Can you work these out from the model? Positions are in its coordinate system, mm. A direction names the side the tool comes from. Give positions to 0.01 mm unless a question says otherwise; leave off trailing zeros. Loops run counter-clockwise (first coordinate to the right, second up) from the corner with the lowest first, then second, coordinate; pieces in that order, holes last. Notation, with made-up numbers: (33, 71.25) -> (65, 71.25) arc R12 ccw to (65, 94.25) -> close; hole circle Ø7 at (53.25, 4.25). An arc over 180 degrees is marked (long way). Use CSV: the item, a comma, the result in double quotes.
from build123d import *

# Parameters (mm, degrees)
BOSS_EXTRUDE4_DEPTH = 13


with BuildPart() as part:
    # Sketch1 → Boss-Extrude4 (new body)
    with BuildSketch(Plane.XY):
        with BuildLine():
            Line((-22, 0), (-32, 0))
            Line((-32, 0), (-32, 4))
            Line((-32, 4), (-24.916186035, 4))
            add(Edge.make_bspline(
                [(24.916186035, 4), (0, 49), (-24.916186035, 4)],
                knots=[3.431344355, 3.431344355, 3.431344355, 5.993433606, 5.993433606, 5.993433606], degree=2, weights=[1, 0.285714286, 1]))
            Line((24.916186035, 4), (32, 4))
            Line((32, 4), (32, 0))
            Line((32, 0), (22, 0))
            add(Edge.make_bspline(
                [(22, 0), (22, 0.432036642), (21.854886362, 1.296109926), (20.997387843, 2.886644647), (19.258004947, 4.669386797), (15.741252168, 6.998785757), (9.364361038, 9.328152259), (0, 10.335923871), (-9.364361038, 9.328152259), (-15.741252168, 6.998785757), (-19.258004947, 4.669386797), (-20.997387843, 2.886644647), (-21.854886362, 1.296109926), (-22, 0.432036642), (-22, 0)],
                knots=[3.141592654, 3.141592654, 3.141592654, 3.141592654, 3.337942194, 3.534291735, 3.730641276, 3.926990817, 4.319689899, 4.71238898, 5.105088062, 5.497787144, 5.694136685, 5.890486225, 6.086835766, 6.283185307, 6.283185307, 6.283185307, 6.283185307], degree=3))
        make_face()
    extrude(amount=BOSS_EXTRUDE4_DEPTH)


solid = part.part
(1) Will these pins go through, and if not, where does the flat tip stop? pin 1 Ø5.5 at (x, z) = (-30, 8.5) entering from +Y; pin 2 Ø1 at (y, z) = (9.5, 10) entering from -X; pin 3 Ø6 at (y, z) = (12.5, 2.5) entering from -X.
Answer sheet:
pin 1,"stops at y = 4"
pin 2,"stops at x = -19.92"
pin 3,"stops at x = -19.1"
(2) If we section it at A-A, the plane x = -26.5: Write out the boundary of the cut face in (y, z), then the cut area to 3 significant figures.
Answer sheet:
outline,"(0, 0) -> (4, 0) -> (4, 13) -> (0, 13) -> close"
area,"52.0 mm2"
(3) If I drill on L1, parallel to Y at x = 25, z = 12.25; L2, parallel to X at y = 7.25, z = 8.5; L3, parallel to X at y = 1.5, z = 11.25, over which ranges is the centre line in solid material (lowest first)? Write a range as from..to.
Answer sheet:
L1,"y = 0..4"
L2,"x = -22.24..-14.67, 14.67..22.24"
L3,"x = -32..-21.69, 21.69..32"
(4) Which directions (+Z, -Z, +X, -X, +Y, -Y) give clear straight access to the entire face, cutting with the end or side of a thin tool? Please do faces 1 (the face through (2.5, 10.1, 13)), 2 (the face through (28, 4, 6)), 3 (the face through (-29, 4, 6)).
Answer sheet:
face 1,"+Z, +X, -X, +Y, -Y"
face 2,"+Z, -Z, +X, +Y"
face 3,"+Z, -Z, -X, +Y"
